```python
from build123d import *

# Parameters (mm, degrees)
BOSS_EXTRUDE1_DEPTH = 76.2
SKETCH2_R           = 18.288
CUT_EXTRUDE1_DEPTH  = 74.93
SKETCH3_W           = 30.896743612
SKETCH3_H           = 8.166199328
CUT_EXTRUDE2_DEPTH  = 55.372
SKETCH5_W           = 22.86
SKETCH5_H           = 42.694539366
CUT_EXTRUDE4_DEPTH  = 55.372
CUT_EXTRUDE5_DEPTH  = 55.372
SKETCH7_R           = 1.5
CUT_EXTRUDE6_DEPTH  = 7.62
FILLET1_R           = 2.54
FILLET2_R           = 2.54
CUT_EXTRUDE7_DEPTH  = 2.54


with BuildPart() as part:
    # Sketch1 → Boss-Extrude1 (new body)
    with BuildSketch(Plane.XY):
        with BuildLine():
            Line((19.05, 38.034196891), (19.05, -25.465803109))
            Line((19.05, -25.465803109), (-20.32, -25.465803109))
            Line((-20.32, -25.465803109), (-20.32, 38.034196891))
            ThreePointArc((-20.32, 38.034196891), (-0.635, 57.719196891), (19.05, 38.034196891))
        make_face()
    extrude(amount=BOSS_EXTRUDE1_DEPTH)

    # Sketch2 → Cut-Extrude1 (cut)
    with BuildSketch(Plane(origin=(0, 0, 0), x_dir=(-1, 0, 0), z_dir=(0, 0, -1))):
        with Locations((0.635, 38.034196891)):
            Circle(SKETCH2_R)
    extrude(amount=-CUT_EXTRUDE1_DEPTH, mode=Mode.SUBTRACT)

    # Sketch3 → Cut-Extrude2 (cut)
    with BuildSketch(Plane.XZ.offset(25.465803109)):
        with Locations((-0.563393949, 67.607273916)):
            Rectangle(SKETCH3_W, SKETCH3_H)
    extrude(amount=-CUT_EXTRUDE2_DEPTH, mode=Mode.SUBTRACT)

    # Sketch5 → Cut-Extrude4 (cut)
    with BuildSketch(Plane.ZY.offset(20.32)):
        with Locations((64.77, -4.118533426)):
            Rectangle(SKETCH5_W, SKETCH5_H)
    extrude(amount=-CUT_EXTRUDE4_DEPTH, mode=Mode.SUBTRACT)

    # Sketch6 → Cut-Extrude5 (cut)
    with BuildSketch(Plane.ZY.offset(20.32)):
        Polygon((49.692334338, 15.234978865), (3.545926494, 15.234978865), (3.545926494, 0), align=None)
        Polygon((49.692334338, 10.776388735), (3.545926494, -4.45859013), (3.545926494, -19.876418407), (49.692334338, -19.876418407), align=None)
    extrude(amount=-CUT_EXTRUDE5_DEPTH, mode=Mode.SUBTRACT)

    # Sketch7 → Cut-Extrude6 (cut)
    with BuildSketch(Plane(origin=(0, -25.465803109, 0), x_dir=(-1, 0, 0), z_dir=(0, -1, 0))):
        with Locations(Location((10.795, -13.97, 0), (0, 0, 90))):
            Circle(SKETCH7_R)
        with Locations(Location((10.795, -39.37, 0), (0, 0, 90))):
            Circle(SKETCH7_R)
        with Locations(Location((-9.525, -13.97, 0), (0, 0, 90))):
            Circle(SKETCH7_R)
        with Locations(Location((-9.525, -39.37, 0), (0, 0, 90))):
            Circle(SKETCH7_R)
    extrude(amount=-CUT_EXTRUDE6_DEPTH, mode=Mode.SUBTRACT)

    # Fillet1
    fillet1_edges = [part.edges().sort_by_distance(p)[0] for p in [
        (-0.635, 17.228736257, 76.2),
    ]]
    fillet(fillet1_edges, radius=FILLET1_R)

    # Fillet2
    fillet2_edges = [part.edges().sort_by_distance(p)[0] for p in [
        (19.05, -4.118533426, 53.34),
        (-20.32, -4.118533426, 53.34),
    ]]
    fillet(fillet2_edges, radius=FILLET2_R)

    # Sketch8 → Cut-Extrude7 (cut)
    with BuildSketch(Plane.ZY.offset(20.32)):
        Polygon((58.58873891, 27.55033505), (62.707128333, 28.447770947), (58.58873891, 29.345907966), (58.58873891, 29.726617101), (63.65925173, 28.62094803), (63.65925173, 28.273892742), (58.58873891, 27.168924793), align=None)
        with BuildLine():
            add(Edge.make_bspline(
                [(64.996431217, 29.322770947), (65.036672351, 29.321620871), (65.114658498, 29.319392057), (65.227191282, 29.304382374), (65.330482027, 29.277639856), (65.409194262, 29.246710575), (65.46543075, 29.217287823), (65.501792779, 29.194596329), (65.532480318, 29.170293168), (65.558238335, 29.145481874), (65.577165676, 29.118219683), (65.591788765, 29.090652513), (65.600610557, 29.061314813), (65.601668573, 29.041210781), (65.602200448, 29.03110428)],
                knots=[0, 0, 0, 0, 1.990507798, 3.857546318, 5.601569732, 7.256660921, 8.027130436, 8.73909373, 9.372800607, 9.961351037, 10.500235976, 11.006911429, 11.500764338, 12, 12, 12, 12], degree=3))
            add(Edge.make_bspline(
                [(65.602200448, 29.03110428), (65.601668573, 29.02099778), (65.600610557, 29.000893748), (65.591788765, 28.971556048), (65.577165676, 28.943988878), (65.558238335, 28.916726687), (65.532480318, 28.891915393), (65.501792779, 28.867612232), (65.46543075, 28.844920738), (65.409194262, 28.815497986), (65.330482027, 28.784568705), (65.227191282, 28.757826187), (65.114658498, 28.742816503), (65.036672351, 28.74058769), (64.996431217, 28.739437614)],
                knots=[0, 0, 0, 0, 0.499235662, 0.993088571, 1.499764024, 2.038648963, 2.627199393, 3.26090627, 3.972869564, 4.743339079, 6.398430268, 8.142453682, 10.009492202, 12, 12, 12, 12], degree=3))
            add(Edge.make_bspline(
                [(64.996431217, 28.739437614), (64.956190084, 28.74058769), (64.878203937, 28.742816503), (64.765671153, 28.757826187), (64.662380408, 28.784568705), (64.583668173, 28.815497986), (64.527431685, 28.844920738), (64.491069656, 28.867612232), (64.460382117, 28.891915393), (64.4346241, 28.916726687), (64.415696759, 28.943988878), (64.401073669, 28.971556048), (64.392251878, 29.000893748), (64.391193862, 29.02099778), (64.390661987, 29.03110428)],
                knots=[0, 0, 0, 0, 1.990507798, 3.857546318, 5.601569732, 7.256660921, 8.027130436, 8.73909373, 9.372800607, 9.961351037, 10.500235976, 11.006911429, 11.500764338, 12, 12, 12, 12], degree=3))
            add(Edge.make_bspline(
                [(64.390661987, 29.03110428), (64.391186666, 29.040981967), (64.392230692, 29.060636942), (64.401235197, 29.089432768), (64.415680324, 29.116822155), (64.434629148, 29.144078002), (64.460380267, 29.168892275), (64.491071648, 29.193190012), (64.52742486, 29.215902902), (64.583786055, 29.245244148), (64.662185902, 29.277227081), (64.765764853, 29.303386129), (64.878127586, 29.319664025), (64.956175178, 29.321713732), (64.996431217, 29.322770947)],
                knots=[0, 0, 0, 0, 0.488404753, 0.971845354, 1.47922561, 2.018860156, 2.608229279, 3.242817664, 3.955771323, 4.727312586, 6.389026247, 8.135475657, 10.006723338, 12, 12, 12, 12], degree=3))
        make_face()
        with BuildLine():
            add(Edge.make_bspline(
                [(64.996431217, 27.258668383), (65.036672351, 27.257518307), (65.114658498, 27.255289493), (65.227191282, 27.24027981), (65.330482027, 27.213537292), (65.409194262, 27.182608011), (65.46543075, 27.153185259), (65.501792779, 27.130493765), (65.532480318, 27.106190604), (65.558238335, 27.08137931), (65.577165676, 27.054117119), (65.591788765, 27.026549949), (65.600610557, 26.997212248), (65.601668573, 26.977108216), (65.602200448, 26.967001716)],
                knots=[0, 0, 0, 0, 1.990507798, 3.857546318, 5.601569732, 7.256660921, 8.027130436, 8.73909373, 9.372800607, 9.961351037, 10.500235976, 11.006911429, 11.500764338, 12, 12, 12, 12], degree=3))
            add(Edge.make_bspline(
                [(65.602200448, 26.967001716), (65.601675763, 26.957124042), (65.600631725, 26.937469089), (65.59162731, 26.908673091), (65.577181819, 26.881284401), (65.558234499, 26.854025675), (65.532477027, 26.829223563), (65.501812643, 26.804874143), (65.465247899, 26.782328727), (65.409537026, 26.751692384), (65.330402294, 26.721274107), (65.227153238, 26.694597501), (65.114719446, 26.678475837), (65.036682016, 26.676403788), (64.996431217, 26.67533505)],
                knots=[0, 0, 0, 0, 0.48835869, 0.971753697, 1.4790861, 2.018669752, 2.607983289, 3.242511825, 3.955398243, 4.732318271, 6.389555434, 8.135840131, 10.00691133, 12, 12, 12, 12], degree=3))
            add(Edge.make_bspline(
                [(64.996431217, 26.67533505), (64.956180419, 26.676403788), (64.878142989, 26.678475837), (64.765709197, 26.694597501), (64.662460141, 26.721274107), (64.583325409, 26.751692384), (64.527614536, 26.782328727), (64.491049792, 26.804874143), (64.460385408, 26.829223563), (64.434627936, 26.854025675), (64.415680616, 26.881284401), (64.401235125, 26.908673091), (64.39223071, 26.937469089), (64.391186672, 26.957124042), (64.390661987, 26.967001716)],
                knots=[0, 0, 0, 0, 1.99308867, 3.864159869, 5.610444566, 7.267681729, 8.044601757, 8.757488175, 9.392016711, 9.981330248, 10.5209139, 11.028246303, 11.51164131, 12, 12, 12, 12], degree=3))
            add(Edge.make_bspline(
                [(64.390661987, 26.967001716), (64.391193862, 26.977108216), (64.392251878, 26.997212248), (64.401073669, 27.026549949), (64.415696759, 27.054117119), (64.4346241, 27.08137931), (64.460382117, 27.106190604), (64.491069656, 27.130493765), (64.527431685, 27.153185259), (64.583668173, 27.182608011), (64.662380408, 27.213537292), (64.765671153, 27.24027981), (64.878203937, 27.255289493), (64.956190084, 27.257518307), (64.996431217, 27.258668383)],
                knots=[0, 0, 0, 0, 0.499235662, 0.993088571, 1.499764024, 2.038648963, 2.627199393, 3.26090627, 3.972869564, 4.743339079, 6.398430268, 8.142453682, 10.009492202, 12, 12, 12, 12], degree=3))
        make_face()
        with BuildLine():
            Line((67.051559423, 25.733027357), (66.243867115, 25.733027357))
            add(Edge.make_bspline(
                [(66.243867115, 25.733027357), (66.28260692, 25.772843106), (66.360174226, 25.852564736), (66.468966307, 25.97888666), (66.572347001, 26.109648304), (66.67019798, 26.244993717), (66.76091061, 26.385954161), (66.846362199, 26.531412433), (66.924350458, 26.682284456), (66.997421295, 26.836864373), (67.0632652, 26.994582281), (67.120200869, 27.154651777), (67.167701253, 27.316032688), (67.207224728, 27.478605836), (67.238213655, 27.642389926), (67.259589839, 27.807443651), (67.273735474, 27.973564747), (67.275188403, 28.084794525), (67.275918397, 28.140679601)],
                knots=[0, 0, 0, 0, 0.992342649, 1.98693169, 2.976855543, 3.969988518, 4.969517551, 5.970693636, 6.982945216, 8.002815687, 9.02486352, 10.035184142, 11.036656235, 12.029148216, 13.02335152, 14.013108037, 15.001727688, 16, 16, 16, 16], degree=3))
            add(Edge.make_bspline(
                [(67.275918397, 28.140679601), (67.275184901, 28.192343133), (67.27372325, 28.295294032), (67.263801037, 28.44878426), (67.246973124, 28.600860245), (67.222920671, 28.751444462), (67.193020341, 28.901036666), (67.155654129, 29.048791927), (67.112174699, 29.195317294), (67.061617766, 29.339705541), (67.006070574, 29.481699791), (66.944044099, 29.619275823), (66.87721261, 29.752732906), (66.806301921, 29.882246985), (66.729139051, 30.006769884), (66.648009526, 30.127575587), (66.561360678, 30.244023811), (66.499211501, 30.317960149), (66.468226089, 30.354822229)],
                knots=[0, 0, 0, 0, 1.030615892, 2.053727828, 3.066966151, 4.081801417, 5.094889563, 6.109178507, 7.121085909, 8.142879786, 9.160153843, 10.161827701, 11.152208124, 12.13713053, 13.106268419, 14.073498001, 15.03951329, 16, 16, 16, 16], degree=3))
            Line((66.468226089, 30.354822229), (67.186174807, 30.354822229))
            add(Edge.make_bspline(
                [(67.186174807, 30.354822229), (67.216874753, 30.319332363), (67.278313081, 30.248308195), (67.365007427, 30.136608354), (67.444835657, 30.019171184), (67.522194874, 29.898457723), (67.593126071, 29.772205249), (67.660248359, 29.641773165), (67.720879773, 29.505913751), (67.777568925, 29.366424056), (67.828739811, 29.223868209), (67.873051444, 29.079290549), (67.909800157, 28.933390224), (67.941592089, 28.786255648), (67.963633891, 28.637172897), (67.98205547, 28.48695015), (67.991590785, 28.33524909), (67.993106473, 28.233705926), (67.993867115, 28.182746909)],
                knots=[0, 0, 0, 0, 0.951172047, 1.903534998, 2.864157892, 3.828872604, 4.809039982, 5.798517374, 6.801478967, 7.823757442, 8.850242752, 9.870807247, 10.887714424, 11.899576751, 12.920723883, 13.941464303, 14.966932353, 16, 16, 16, 16], degree=3))
            add(Edge.make_bspline(
                [(67.993867115, 28.182746909), (67.993320557, 28.127802038), (67.992230776, 28.018247462), (67.979500696, 27.854750164), (67.960602263, 27.692433158), (67.935061158, 27.530830321), (67.900126876, 27.370310002), (67.859101093, 27.210379802), (67.809895139, 27.051761284), (67.752895083, 26.894698646), (67.689344878, 26.739587526), (67.619078904, 26.586642874), (67.541299534, 26.437089331), (67.456857335, 26.29034603), (67.366560774, 26.146022013), (67.26796876, 26.005539052), (67.163825129, 25.866798877), (67.089134493, 25.777800373), (67.051559423, 25.733027357)],
                knots=[0, 0, 0, 0, 0.983526716, 1.961053866, 2.934201006, 3.908957034, 4.888845537, 5.874284043, 6.864251573, 7.860925746, 8.864846135, 9.864607242, 10.873329523, 11.881739335, 12.895214845, 13.920156785, 14.953680705, 16, 16, 16, 16], degree=3))
        make_face()
    extrude(amount=-CUT_EXTRUDE7_DEPTH, mode=Mode.SUBTRACT)


solid = part.part
```
CAD build for the part. Positions are in the model's coordinates, mm. A direction names the side the tool comes from. Give positions to 0.01 mm unless a question says otherwise; leave off trailing zeros. Write each loop counter-clockwise with the first axis right and the second up, starting at its lowest first coordinate (ties: lowest second). Pieces come first, ordered by that corner, then holes. Notation, with made-up numbers: (-31.5, 10) -> (10.5, 10) arc R15 ccw to (10.5, 22) -> close; hole circle Ø8 at (5, 49). An arc over 180 degrees is marked (long way). Write each question's results on one line, items separated by ' | '.
1. Which spindle directions (+Z, -Z, +X, -X, +Y, -Y) get a long thin tool onto all of the face, cutting with end or side? Do faces 4 (the cylindrical face through (10.539, -22.71, 15.076)), 5 (the flat face through (0, -2, 0)), 6 (the cylindrical face through (1.746, 56.167, 36.94)), 7 (the flat face through (-0.911, 7.511, 26.296)), 8 (the flat face through (-19.068, 27.993, 60.619)). Say none if no direction does.
Geometry check:
face 4: -Y | face 5: -Z, +X, -X, +Y, -Y | face 6: -Z | face 7: +X, -X | face 8: -X
2. Cut at C-C, the plane z = 55.5. Write the cut outline in (x, y) (3 decimals).
Geometry check:
outline: (-20.32, 17.229) -> (19.05, 17.229) -> (19.05, 38.034) arc R19.685 ccw to (-20.32, 38.034) -> close; hole circle Ø36.576 at (-0.635, 38.034)
3. Two-plate mould, pull along X, no slides. Class faces 1 (the cylindrical face through (-0.359, 17.993, 75.476)), 2 (the flat face through (-17.78, 29, 61)), 3 (the cylindrical face through (8.95, -22.71, 37.984)): pulls with the +X half, pulls with the -X half, needs draft (parallel to the pull), parting line crosses it, or undercut.
Geometry check:
face 1: needs draft | face 2: pulls with the -X half | face 3: undercut
4. Cut at A-A, the plane x = 5. Write the cut outline in (y, z).
Geometry check:
outline: (-25.47, 0) -> (20.64, 0) -> (20.64, 63.52) -> (17.23, 63.52) -> (17.23, 53.34) -> (-25.47, 53.34) -> close; (17.23, 71.69) -> (20.64, 71.69) -> (20.64, 74.93) -> (55.43, 74.93) -> (55.43, 0) -> (56.9, 0) -> (56.9, 76.2) -> (19.77, 76.2) arc R2.54 ccw to (17.23, 73.66) -> close; hole (-19.88, 3.55) -> (-4.46, 3.55) -> (10.78, 49.69) -> (-19.88, 49.69) -> close; hole (0, 3.55) -> (15.23, 3.55) -> (15.23, 49.69) -> close
5. Cut at D-D, the plane y = 42. Write the cut outline in (x, z), then the cut area to 3 significant figures.
Geometry check:
outline: (-19.92, 0) -> (-18.49, 0) -> (-18.49, 74.93) -> (17.22, 74.93) -> (17.22, 0) -> (18.65, 0) -> (18.65, 76.2) -> (-19.92, 76.2) -> close | area: 263 mm²
6. Wall check: probe 1 along X at (y, z) = (-24.3, 39.37) (3 decimals); probe 2 along Y at (x, z) = (-4, 46.5). Give the ranges that are in metal, low to high. Write a range as [from, to].
Geometry check:
probe 1: [-20.32, -12.295], [-9.295, 8.025], [11.025, 19.05] | probe 2: [-25.47, -19.88], [9.72, 14.18], [15.23, 20.06], [56.01, 57.43]
7. Drop flat-ended pins along their axis: P1, Ø1.5, axis at x = -6, y = 14.5, coming from the +Z side; P2, Ø2.5, axis at x = -10.795, z = 13.97, coming from the +Y side; P3, Ø0.9, axis at x = -19, z = 66.5, coming from the +Y side. Give the stop position or say it passes through.
Geometry check:
P1: z = 53.34 | P2: y = 55.59 | P3: y = 46.19
8. Cut at B-B, the plane z = 39.37. Write the cut outline in (x, y) (3 decimals), then the cut area to 3 significant figures.
Geometry check:
outline: (-20.32, -25.466) -> (-12.295, -25.466) -> (-12.295, -19.876) -> (-20.32, -19.876) -> close; (-20.32, 7.369) -> (19.05, 7.369) -> (19.05, 11.827) -> (-20.32, 11.827) -> close; (-20.32, 15.235) -> (19.05, 15.235) -> (19.05, 38.034) arc R19.685 ccw to (-20.32, 38.034) -> close; (-9.295, -25.466) -> (8.025, -25.466) -> (8.025, -19.876) -> (-9.295, -19.876) -> close; (11.025, -25.466) -> (19.05, -25.466) -> (19.05, -19.876) -> (11.025, -19.876) -> close; hole circle Ø36.576 at (-0.635, 38.034) | area: 818 mm²
